from build123d import *

# Parameters (mm, degrees)
BOSS_EXTRUDE1_DEPTH     = 43
CUT_EXTRUDE6_DEPTH      = 74.561199011
CUT_EXTRUDE6_DEPTH_BACK = 74.561199011
SKETCH8_R               = 1.6383
SKETCH15_W              = 10.528106576
SKETCH15_H              = 16
BOSS_EXTRUDE2_DEPTH     = 20
CUT_EXTRUDE7_DEPTH      = 74.561199011
CUT_EXTRUDE7_DEPTH_BACK = 74.561199011
SKETCH16_R              = 2.5
FILLET5_SIZE            = 2
FILLET6_SIZE            = 2
CUT_EXTRUDE8_DEPTH      = 3.5
FILLET7_R               = 0.5
FILLET8_R               = 0.5
CUT_EXTRUDE9_DEPTH      = 74.561199011
CUT_EXTRUDE9_DEPTH_BACK = 74.561199011
FILLET9_R               = 5


with BuildPart() as part:
    # Sketch1 → Boss-Extrude1 (new body)
    with BuildSketch(Plane(origin=(0, 0, 0), x_dir=(0, 0, -1), z_dir=(1, 0, 0))):
        Polygon((-50, 0), (0, 0), (0, -11), (7.5, -11), (7.5, -16), (-57.5, -16), (-57.5, -11), (-50, -11), align=None)
    extrude(amount=BOSS_EXTRUDE1_DEPTH)

    # Sketch8 → Cut-Extrude6 (cut, two sides: drawn at the far end of the back side and taken through both)
    with BuildSketch(Plane(origin=(0, 0, 0), x_dir=(1, 0, 0), z_dir=(0, 1, 0)).offset(-CUT_EXTRUDE6_DEPTH_BACK)):
        with Locations(Location((8.307443012, -40, 0), (0, 0, 270))):
            Circle(SKETCH8_R)
        with Locations(Location((8.307443012, -10, 0), (0, 0, 270))):
            Circle(SKETCH8_R)
    extrude(amount=CUT_EXTRUDE6_DEPTH + CUT_EXTRUDE6_DEPTH_BACK, mode=Mode.SUBTRACT)

    # Sketch15 → Boss-Extrude2 (add)
    with BuildSketch(Plane.ZY):
        with Locations((42, -8)):
            Rectangle(SKETCH15_W, SKETCH15_H)
        with Locations((8, -8)):
            Rectangle(SKETCH15_W, SKETCH15_H)
    extrude(amount=BOSS_EXTRUDE2_DEPTH)

    # Sketch16 → Cut-Extrude7 (cut, two sides: drawn at the far end of the back side and taken through both)
    with BuildSketch(Plane(origin=(0, 0, 0), x_dir=(1, 0, 0), z_dir=(0, 1, 0)).offset(-CUT_EXTRUDE7_DEPTH_BACK)):
        with Locations(Location((-14.585283135, -8, 0), (0, 0, 270))):
            Circle(SKETCH16_R)
        with Locations(Location((-14.585283135, -42, 0), (0, 0, 90))):
            Circle(SKETCH16_R)
    extrude(amount=CUT_EXTRUDE7_DEPTH + CUT_EXTRUDE7_DEPTH_BACK, mode=Mode.SUBTRACT)

    # Fillet5
    # a fillet whose section is not a circle: 2 mm, written as the material it takes off along each edge
    with BuildSketch(Plane(origin=(-14.585283135, 0, 8), x_dir=(0, 0, 1), z_dir=(-1, 0, 0))) as fillet5_piece_1:
        with BuildLine():
            Bezier((2.5 + FILLET5_SIZE, 0), (2.5, 0), (2.5, -FILLET5_SIZE), weights=[1, 0.141421356, 1])
            Line((2.5, -FILLET5_SIZE), (2.5, 0))
            Line((2.5, 0), (2.5 + FILLET5_SIZE, 0))
        make_face()
    revolve(axis=Axis((-14.585283135, 0, 8), (0, 1, 0)), mode=Mode.SUBTRACT)

    # Fillet6
    # a fillet whose section is not a circle: 2 mm, written as the material it takes off along each edge
    with BuildSketch(Plane(origin=(-14.585283135, 0, 42), x_dir=(0, 0, -1), z_dir=(1, 0, 0))) as fillet6_piece_1:
        with BuildLine():
            Bezier((2.5 + FILLET6_SIZE, 0), (2.5, 0), (2.5, -FILLET6_SIZE), weights=[1, 0.141421356, 1])
            Line((2.5, -FILLET6_SIZE), (2.5, 0))
            Line((2.5, 0), (2.5 + FILLET6_SIZE, 0))
        make_face()
    revolve(axis=Axis((-14.585283135, 0, 42), (0, 1, 0)), mode=Mode.SUBTRACT)

    # Sketch20 → Cut-Extrude8 (cut)
    with BuildSketch(Plane.XZ.offset(16)):
        Polygon((13.503595435, 10), (10.905519224, 14.5), (5.709366801, 14.5), (3.11129059, 10), (5.709366801, 5.5), (10.905519224, 5.5), align=None)
        Polygon((10.905519224, 44.5), (13.503595435, 40), (10.905519224, 35.5), (5.709366801, 35.5), (3.11129059, 40), (5.709366801, 44.5), align=None)
    extrude(amount=-CUT_EXTRUDE8_DEPTH, mode=Mode.SUBTRACT)

    # Fillet7
    fillet7_edges = [part.edges().sort_by_distance(p)[0] for p in [
        (12.204557329, -16, 7.75),
        (12.204557329, -16, 12.25),
        (8.307443012, -16, 14.5),
        (4.410328695, -16, 12.25),
        (4.410328695, -16, 7.75),
        (8.307443012, -16, 5.5),
    ]]
    fillet(fillet7_edges, radius=FILLET7_R)

    # Fillet8
    fillet8_edges = [part.edges().sort_by_distance(p)[0] for p in [
        (8.307443012, -16, 44.5),
        (4.410328695, -16, 42.25),
        (4.410328695, -16, 37.75),
        (8.307443012, -16, 35.5),
        (12.204557329, -16, 37.75),
        (12.204557329, -16, 42.25),
    ]]
    fillet(fillet8_edges, radius=FILLET8_R)

    # Sketch21 → Cut-Extrude9 (cut, two sides: drawn at the far end of the back side and taken through both)
    with BuildSketch(Plane(origin=(0, 0, 0), x_dir=(1, 0, 0), z_dir=(0, 1, 0)).offset(-CUT_EXTRUDE9_DEPTH_BACK)):
        Polygon((16.186241981, -25), (16.186241981, -8.3617), (36, -8.3617), (36, -40), (16.186241981, -40), align=None)
    extrude(amount=CUT_EXTRUDE9_DEPTH + CUT_EXTRUDE9_DEPTH_BACK, mode=Mode.SUBTRACT)

    # Fillet9
    # the kernel refuses this fillet: 5 mm, written as the material it takes off along each edge
    with BuildSketch(Plane(origin=(-30, 0, 50), x_dir=(0, 0, -1), z_dir=(1, 0, 0)), Plane(origin=(-30, 0, 0), x_dir=(0, -1, 0), z_dir=(1, 0, 0))) as fillet9_piece_1:
        with BuildLine():
            CenterArc((FILLET9_R, -FILLET9_R), FILLET9_R, 90, 90)
            Line((0, -FILLET9_R), (-FILLET9_R * 0.02, -FILLET9_R))
            Line((-FILLET9_R * 0.02, -FILLET9_R), (-FILLET9_R * 0.02, FILLET9_R * 0.02))
            Line((-FILLET9_R * 0.02, FILLET9_R * 0.02), (FILLET9_R, FILLET9_R * 0.02))
            Line((FILLET9_R, FILLET9_R * 0.02), (FILLET9_R, 0))
        make_face()
    extrude(amount=103, mode=Mode.SUBTRACT)


solid = part.part
Can you work these out from the model? Positions are in its coordinate system, mm. A direction names the side the tool comes from. Give positions to 0.01 mm unless a question says otherwise; leave off trailing zeros. Order: outer loops, then holes, each group sorted by start corner. A loop starts at its lowest first (then second) coordinate and runs counter-clockwise, first axis right, second up. Notation, with made-up numbers: M 58.5,81 L 106.5,81 A21 cw 106.5,90 Z; hole C 24.25,-4 d8. An arc over 180 degrees is marked long. One line per question, with ' | ' between items.
Item 1: Suppose I cut it at A-A, the plane x = 32. Write out the boundary of the cut face in (y, z).
Answer block:
outline: M -16,-7.5 L -11,-7.5 L -11,0 L -5,0 A5 ccw 0,5 L 0,8.36 L -16,8.36 Z; M -16,40 L 0,40 L 0,45 A5 ccw -5,50 L -11,50 L -11,57.5 L -16,57.5 Z
Item 2: Please list where these lines run through material, in increasing order: L1, parallel to X at y = -4.5, z = 14; L2, parallel to Z at x = 24.5, y = -5.75; L3, parallel to Z at x = 6, y = -12.75.
Answer block:
L1: x = 0 to 16.19, 36 to 43 | L2: z = 0 to 8.36, 40 to 50 | L3: z = -7.5 to 5.5, 14.5 to 35.5, 44.5 to 57.5
Item 3: Suppose I cut it at C-C, the plane y = -14.5. Give the number of separate pieces and of enclosed holes in the cut face, then the cut area to 3 significant figures.
Answer block:
separate pieces: 1 | enclosed holes: 5 | area: 2,410 mm2
Item 4: Suppose I cut it at B-B, the plane z = 31. Write out the boundary of the cut face in (x, y).
Answer block:
outline: M 0,-16 L 16.19,-16 L 16.19,0 L 0,0 Z; M 36,-16 L 43,-16 L 43,0 L 36,0 Z
Item 5: We'd pull the mould along Z, two halves only. Please class faces 6 (the face through (-10, -8, 36.736)), 7 (the face through (-20, -8, 8)), 8 (the face through (21, -13, -7.5)): released by +Z, released by -Z, zero draft, split by the parting line, or undercut.
Answer block:
face 6: undercut | face 7: zero draft | face 8: released by -Z
Item 6: For faces 1 (the face through (21, -11, -4)), 2 (the face through (8, -14, 5.5)), 3 (the face through (16.186, -8, 24)), 4 (the face through (11, -16, 25)), 5 (the face through (21, -8, 50)), which set-ups out of +Z, -Z, +X, -X, +Y, -Y let a thin tool reach every point of the face, with its end or its side?
Answer block:
face 1: -Z, +X, -X, +Y | face 2: -Y | face 3: +Y, -Y | face 4: +Z, -Z, +X, -X, -Y | face 5: +Z, +X, -X, +Y
Item 7: I'm going to push flat-ended pins straight in: pin 1 Ø4.5 at (x, z) = (-14.59, 8) entering from -Y; pin 2 Ø6 at (x, z) = (28, -0.5) entering from +Y; pin 3 Ø6 at (x, y) = (35, -6.5) entering from +Z; pin 4 Ø5 at (x, y) = (24.5, -4) entering from -Z. Where does each tip first touch, or does it pass through?
Answer block:
pin 1: passes through | pin 2: stops at y = -0.67 | pin 3: stops at z = 50 | pin 4: stops at z = 0
Item 8: Suppose I cut it at D-D, the plane y = -8. Write out the boundary of the cut face in (x, z).
Answer block:
outline: M -20,2.74 L 0,2.74 L 0,0 L 43,0 L 43,50 L 0,50 L 0,47.26 L -20,47.26 L -20,36.74 L 0,36.74 L 0,13.26 L -20,13.26 Z; hole C -14.59,8 d5; hole C -14.59,42 d5; hole C 8.31,10 d3.28; hole C 8.31,40 d3.28; hole M 16.19,8.36 L 36,8.36 L 36,40 L 16.19,40 Z
